Here's how the part is built. I have some questions about the finished solid (model axes, mm). A direction names the side the tool comes from. Round coordinates to 2 decimals unless told otherwise and drop trailing zeros. Answer as CSV lines item,"result".
Autodesk Fusion 360 part; units mm, degrees
sketch "Sketch1" plane through (0, 0, 0) normal (0, 1, 0) x (1, 0, 0)
  line L0 (7.6, 7.5) -> (-7.6, 7.5)
  line L1 (-7.6, 7.5) -> (-7.6, -7.5)
  line L2 (-7.6, -7.5) -> (7.6, -7.5)
  line L3 (7.6, -7.5) -> (7.6, 7.5)
  line L4 (7.6, 7.5) -> (-7.6, -7.5) construction
  line L5 (-7.6, 7.5) -> (7.6, -7.5) construction
  line L6 (7.6, -192) -> (-7.6, -192)
  line L7 (-7.6, -192) -> (-7.6, -207)
  line L8 (-7.6, -207) -> (7.6, -207)
  line L9 (7.6, -207) -> (7.6, -192)
  line L10 (7.6, -192) -> (-7.6, -207) construction
  line L11 (-7.6, -192) -> (7.6, -207) construction
  circle A0 centre (0, -174.75) radius 1.6
  circle A1 centre (0, -99.75) radius 1.6
  circle A2 centre (0, -24.75) radius 1.6
  line L12 (12.6, -207) -> (-12.6, -207)
  line L13 (-12.6, -207) -> (-12.6, 7.5)
  line L14 (-12.6, 7.5) -> (12.6, 7.5)
  line L15 (12.6, 7.5) -> (12.6, -207)
  line L16 (12.6, -207) -> (-12.6, 7.5) construction
  line L17 (-12.6, -207) -> (12.6, 7.5) construction
  point P0 (0, -199.5)
  point P1 (0, -99.75)
  dimension "d1" = 15.2
  dimension "d2" = 15
  dimension "d3" = 15.2
  dimension "d4" = 15
  dimension "d5" = 184.5
  dimension "d6" = 3.2
  dimension "d12" = 0
  dimension "d13" = 150
  dimension "d14" = 25.2
  dimension "d20" = 207
extrude "Extrude1" add sketch "Sketch1" along normal blind 7 contours L1 L2 L3 L6 L7 L9 L12 L13 L14 L15
fillet "Fillet1" radius 2 2 edges at (-12.6, 0, 99.75) (12.6, 0, 99.75)
move_face "OffsetFaces1" offset -0.1 3 faces at (-7.6, 2.3333, 197) (7.6, 2.3333, 202) (2.5333, 2.3333, 192)
move_face "OffsetFaces2" offset -0.1 3 faces at (-2.5333, 2.3333, 7.5) (-7.6, 2.3333, -2.5) (7.6, 2.3333, 2.5)
chamfer "Chamfer1" distance 0.4 angle 45 1 faces at (0, 7, 12.7833)
equation "d14 = 15.2 mm + 10 mm"
1. If I drill on line 1 (Z direction, x = 0, y = 1.5); line 2 (X direction, y = 5, z = 99.75); line 3 (Z direction, x = -2.25, y = 2), over which ranges is the centre line in solid material (lowest first)?
Numbers:
line 1,"z = 7.6 to 23.15, 26.35 to 98.15, 101.35 to 173.15, 176.35 to 191.9"
line 2,"x = -12.6 to -1.6, 1.6 to 12.6"
line 3,"z = 7.6 to 191.9"
2. For pin 1 Ø3.5 at (x, z) = (0, 24.75) entering from +Y; pin 2 Ø4 at (x, z) = (1, 14.5) entering from -Y; pin 3 Ø3 at (x, y) = (-2.5, 5) entering from -Z; pin 4 Ø1.5 at (x, y) = (-4, 1) entering from +Z, each with a flat end and sliding along its axis, tell me the tip position at first contact or that it passes through.
Numbers:
pin 1,"stops at y = 6.75"
pin 2,"stops at y = 0"
pin 3,"stops at z = 7.6"
pin 4,"stops at z = 191.9"
3. On a 3-axis mill with a long thin cutter (end or side, diameter ignored), from which of +Z, -Z, +X, -X, +Y, -Y can I reach the whole of each face in a straight line? I mean faces 1 (the face through (-10, 3, 207)), 2 (the face through (7.7, 3, 0)), 3 (the face through (0, 3, 191.9)). Say none if no direction works.
Numbers:
face 1,"+Z, +X, -X, +Y, -Y"
face 2,"-Z, +Y, -Y"
face 3,"+Z, +Y, -Y"
